from build123d import *

# Parameters (mm, degrees)
F0_W      = 25.4
F0_H      = 25.4
F1_DEPTH  = 6.35
F3_DEPTH  = 25.4
F4_DEPTH  = 25.4
F2_W      = 1.5741327426
F2_H      = 1.3268706389
F2_W_2    = 1.187200658
F2_H_2    = 1.2226499384
F5_DEPTH  = 25.4
F6_DEPTH  = 25.4
F7_DEPTH  = 25.4
F8_DEPTH  = 25.4
F9_DEPTH  = 25.4
F10_DEPTH = 25.4
F2_W_3    = 0.0468016022
F2_H_3    = 2.728624735
F11_DEPTH = 25.4


with BuildPart() as f1:
    # F0 (on Front) → F1 (new body)
    with BuildSketch(Plane.XZ):
        with Locations((12.7, 12.7)):
            Rectangle(F0_W, F0_H)
    extrude(amount=F1_DEPTH)

    # F2 (on face) → F3 (cut)
    with BuildSketch(Plane.XZ.offset(6.35)):
        Polygon((11.3045458782, 12.6861063085), (11.2601406232, 12.6359642364), (11.3882992748, 11.9951701235), (11.4073375334, 11.9818783017), (11.4946379989, 12.0078130807), (11.3568859374, 12.6965743064), align=None)
    extrude(amount=-F3_DEPTH, mode=Mode.SUBTRACT)

    # F2 (on face) → F4 (cut)
    with BuildSketch(Plane.XZ.offset(6.35)):
        Polygon((4.8667113453, 19.705099985), (4.1047113453, 19.705099985), (4.1047113453, 16.530099985), (4.8667113453, 16.530099985), (4.8667113453, 17.646435377), (6.1755171202, 16.4531112731), (6.6484752777, 17.0069300941), (5.8113521077, 17.7406859724), (6.6484752777, 18.6957382214), (5.7038345153, 19.5237355067), (4.8667113453, 18.5686832578), align=None)
        Polygon((17.3532462063, 20.0170688259), (16.7224295437, 19.5896178484), (18.3006953448, 17.5494197756), (16.1248423702, 15.4179709552), (16.7738881073, 14.7554037454), (21.310064048, 19.1990067695), (20.8210359426, 19.650104071), (18.7980631883, 18.1141414298), align=None)
        Polygon((9.8554994911, 19.5896178484), (9.8554994911, 17.7037799731), (9.8554994911, 15.278255567), (11.8336537853, 15.278255567), (11.8336537853, 16.040255567), (10.5636537853, 16.040255567), (10.5636537853, 16.802255567), (11.1025738376, 16.802255567), (11.1025738376, 18.0656178484), (10.5251594293, 18.0656178484), (10.5251594293, 18.8276178484), (11.7951594293, 18.8276178484), (11.7951594293, 19.5896178484), align=None)
    extrude(amount=-F4_DEPTH, mode=Mode.SUBTRACT)

    # F2 (on face) → F5 (cut)
    with BuildSketch(Plane.XZ.offset(6.35)):
        Polygon((11.3918762654, 11.963872239), (11.3760931417, 11.9772851467), (10.3443460539, 11.9772851467), (10.3443460539, 10.6504149735), (11.3918762654, 10.6504149735), align=None)
        Polygon((10.3443460539, 6.4602969214), (11.3918762654, 6.4602969214), (11.3918762654, 6.5283267759), (11.3918762654, 7.2983205318), (10.3443460539, 7.2983205318), (10.3443460539, 6.5283267759), align=None)
        with Locations((12.4582835298, 4.6096618753)):
            Rectangle(F2_W, F2_H)
        with Locations((11.3569586538, 0.6113249692)):
            Rectangle(F2_W_2, F2_H_2)
        Polygon((11.3918762654, 10.0218970329), (10.3443460539, 10.0218970329), (10.3443460539, 9.8811993375), (10.3443460539, 9.4632143155), (11.3918762654, 9.4632143155), align=None)
    extrude(amount=-F5_DEPTH, mode=Mode.SUBTRACT)

    # F2 (on face) → F6 (cut)
    with BuildSketch(Plane.XZ.offset(6.35)):
        Polygon((12.4394055456, 6.4602969214), (13.2453499011, 6.4602969214), (12.4394055456, 8.1363441423), (11.3918762654, 8.1363441423), (12.396886896, 6.5283267759), align=None)
        Polygon((12.4394055456, 8.1363441423), (13.2453499011, 6.4602969214), (13.2194478065, 10.0218970329), (12.4394055456, 10.0218970329), align=None)
    extrude(amount=-F6_DEPTH, mode=Mode.SUBTRACT)

    # F2 (on face) → F7 (cut)
    with BuildSketch(Plane.XZ.offset(6.35)):
        Polygon((10.3443460539, 8.6950268596), (10.3443460539, 8.1466408446), (10.3525146842, 8.1363441423), (11.3799376413, 8.1363441423), (11.3918762654, 8.1456918269), (11.3918762654, 8.6950268596), align=None)
        Polygon((11.3918762654, 10.63934993), (11.3918762654, 10.0235464051), (11.3941496238, 10.0218970329), (12.4334173265, 10.0218970329), (12.4350024447, 10.0245388949), (11.3967579036, 10.6474859888), align=None)
    extrude(amount=-F7_DEPTH, mode=Mode.SUBTRACT)

    # F2 (on face) → F8 (cut)
    with BuildSketch(Plane.XZ.offset(6.35)):
        Polygon((0, 22.8981861721), (5.8363882299, 25.4), (0, 25.4), align=None)
        Polygon((25.4, 25.4), (20.1304874707, 25.4), (25.4, 21.8567334698), align=None)
        Polygon((4.8287836991, 13.6944320588), (0, 17.8181861721), (0, 0), (9.3666529283, 0), (9.3666529283, 2.728624735), (13.2070397958, 2.728624735), (13.2453499011, 2.7803417761), (13.2453499011, 2.8986970428), (9.3666529283, 2.8986970428), (9.3666529283, 3.9462265559), (10.553852655, 3.9462265559), (10.553852655, 5.2730971947), (9.3666529283, 5.2730971947), (9.3666529283, 6.3206264749), (9.3993271689, 6.3813072698), (10.3443460539, 8.1363441423), (9.3666529283, 8.1363441423), (9.3666529283, 9.8811993375), (10.3443460539, 9.8811993375), (10.3443460539, 10.0218970329), (9.3666529283, 10.0218970329), (9.3666529283, 12.6756383106), (11.1529044807, 12.6756383106), (11.2522058189, 12.7877686173), (11.2522058189, 13.6944320588), align=None)
        Polygon((16.1153711372, 23.9690360215), (8.5006434467, 23.6856243072), (2.7146538465, 21.0693627863), (21.7646538465, 21.0693627863), align=None)
        Polygon((25.4, 0), (25.4, 16.7767334698), (20.1682399362, 13.1779577565), (16.3582399362, 13.1779577565), (16.3582399362, 1.7479577565), (14.5153499011, 0), align=None)
    extrude(amount=-F8_DEPTH, mode=Mode.SUBTRACT)

    # F2 (on face) → F9 (cut)
    with BuildSketch(Plane.XZ.offset(6.35)):
        Polygon((10.3443460539, 6.5283267759), (9.3993271689, 6.3813072698), (9.3666529283, 6.3206264749), (10.3443460539, 6.4602969214), align=None)
        Polygon((11.3918762654, 6.4602969214), (12.4394055456, 6.4602969214), (12.396886896, 6.5283267759), (11.3918762654, 6.5283267759), align=None)
    extrude(amount=-F9_DEPTH, mode=Mode.SUBTRACT)

    # F2 (on face) → F10 (cut)
    with BuildSketch(Plane.XZ.offset(6.35)):
        Polygon((11.2931728363, 7.9554002732), (10.4726087302, 7.9641295597), (10.2478063918, 7.5466390744), (11.5114087239, 7.5466390744), align=None)
    extrude(amount=-F10_DEPTH, mode=Mode.SUBTRACT)

    # F2 (on face) → F11 (cut)
    with BuildSketch(Plane.XZ.offset(6.35)):
        with Locations((13.2687507022, 1.3643123675)):
            Rectangle(F2_W_3, F2_H_3)
    extrude(amount=-F11_DEPTH, mode=Mode.SUBTRACT)


solid = f1.part
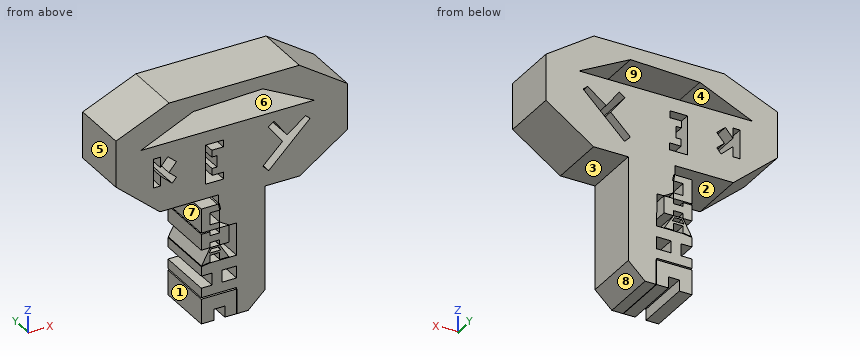
Could you check a few things on this model? Use its own coordinates, in mm. Face numbers are marked on the shaded views. A direction names the side the tool comes from. Coordinates: 2 decimals unless noted, no trailing zeros. Order: outer loops, then holes, each group sorted by start corner. A loop starts at its lowest first (then second) coordinate and runs counter-clockwise, first axis right, second up. Notation, with made-up numbers: (9.25, 61.25) -> (24.25, 61.25) arc R15 ccw to (24.25, 78.25) -> close; hole circle Ø1 at (67, -21). An arc over 180 degrees is marked (long way). One line per item, written item: value. Start each with the question number.
1) Imagine slicing it at D-D on x = 7.5. List the corners of the cut face in (y, z) for me, plus the area to 3 significant figures.
2) Imagine slicing it at C-C on x = 19.5. List the corners of the cut face in (y, z) for me.
3) We'd pull the mould along Z, two halves only. Please class the marked faces 6, 7, 8 and 9: +Z half, -Z half, draft (parallel to the pull), parting line (faces both ways), or undercut.
4) I'm going to push flat-ended pins straight in: pin 1 (3 mm diameter, centred on y = -5.5, z = 6, fed in from +X); pin 2 (1 mm diameter, centred on x = 7, z = 7.5, fed in from -Y); pin 3 (1 mm diameter, centred on y = -2.5, z = 1, fed in from +X); pin 4 (3 mm diameter, centred on y = -3, z = 8.5, fed in from -X). Where does each tip first touch, or does it pass through?
5) If I drill on L1, parallel to X at y = -5.5, z = 4.25; L2, parallel to Z at x = 13, y = -3.75; L3, parallel to Z at x = 6.25, y = -4.25, over which ranges is the centre line in solid material (lowest first)? Write a range as [from, to].
6) Imagine slicing it at A-A on x = 15. List the corners of the cut face in (y, z) for me, plus the area to 3 significant figures.
7) Imagine slicing it at B-B on y = -2.25. Count the separate pieces of the cut face and the enclosed holes in it, plus the area to 3 significant figures.
8) Which directions (+Z, -Z, +X, -X, +Y, -Y) give clear straight access to the entire face, cutting with the end or side of a thin tool? Please do the marked faces 1, 2, 3, 4 and 5.
Answer list:
1. outline: (-6.35, 13.69) -> (0, 13.69) -> (0, 21.07) -> (-6.35, 21.07) -> close; (-6.35, 23.23) -> (0, 23.23) -> (0, 25.4) -> (-6.35, 25.4) -> close
1. area: 60.6 mm2
2. outline: (-6.35, 13.18) -> (0, 13.18) -> (0, 17.43) -> (-6.35, 17.43) -> close; (-6.35, 18.65) -> (0, 18.65) -> (0, 21.07) -> (-6.35, 21.07) -> close; (-6.35, 22.23) -> (0, 22.23) -> (0, 25.4) -> (-6.35, 25.4) -> close
3. face 6: undercut
3. face 7: draft
3. face 8: -Z half
3. face 9: undercut
4. pin 1: stops at x = 16.36
4. pin 2: passes through
4. pin 3: stops at x = 16.1
4. pin 4: stops at x = 9.37
5. L1: x = [10.55, 11.67], [13.25, 16.36]
5. L2: z = [0, 2.73], [2.9, 3.95], [5.27, 6.46], [10.02, 21.07], [23.85, 25.4]
5. L3: z = [13.69, 16.54], [17.36, 18.24], [19.05, 21.07], [22.67, 25.4]
6. outline: (-6.35, 0.46) -> (0, 0.46) -> (0, 21.07) -> (-6.35, 21.07) -> close; (-6.35, 23.93) -> (0, 23.93) -> (0, 25.4) -> (-6.35, 25.4) -> close
6. area: 140 mm2
7. separate pieces: 1
7. enclosed holes: 10
7. area: 288 mm2
8. face 1: -Z, -X, +Y, -Y
8. face 2: -X, +Y, -Y
8. face 3: -Z, +X, +Y, -Y
8. face 4: +Y, -Y
8. face 5: +Z, -Z, -X, +Y, -Y
